Source: CAD feature listing. Evaluate the final solid. Frame: model axes, mm. Face numbers are marked on the shaded views. A direction names the side the tool comes from. Coordinates: 2 decimals unless noted, no trailing zeros. Write each loop counter-clockwise with the first axis right and the second up, starting at its lowest first coordinate (ties: lowest second). Pieces come first, ordered by that corner, then holes. Notation, with made-up numbers: (-8.75, 38) - (15.25, 38) arc R25 ccw to (15.25, 54) - close; hole circle Ø6 at (18, 0.5). An arc over 180 degrees is marked (long way). One line per item, written item: value.
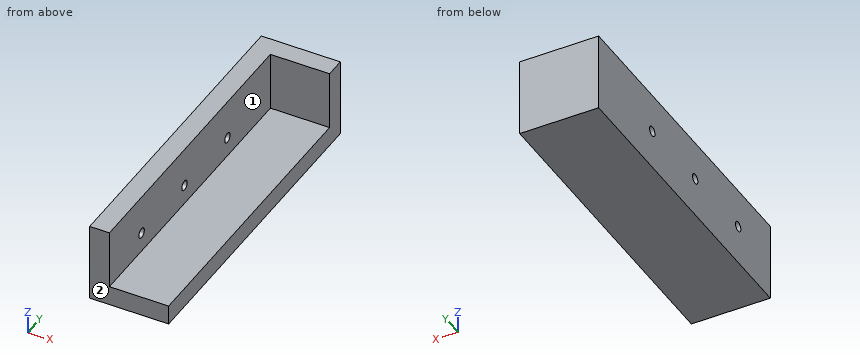
from build123d import *

# Parameters (mm, degrees)
F1_DEPTH = 101.6
F2_W     = 25.4
F2_H     = 25.4
F3_DEPTH = 6.35
F4_R     = 1.5875
F5_DEPTH = 25.4


with BuildPart() as f1:
    # F0 (on Front) → F1 (new body)
    with BuildSketch(Plane.XZ):
        Polygon((0, 25.4), (0, 0), (25.4, 0), (25.4, 6.35), (6.35, 6.35), (6.35, 25.4), align=None)
    extrude(amount=F1_DEPTH)

    # F2 (on Front) → F3 (join)
    with BuildSketch(Plane.XZ):
        with Locations((12.7, 12.7)):
            Rectangle(F2_W, F2_H)
    extrude(amount=F3_DEPTH)

    # F4 (on face) → F5 (cut)
    with BuildSketch(Plane.YZ.offset(6.35)):
        with Locations((-31.75, 12.7)):
            Circle(F4_R)
        with Locations((-57.15, 12.7)):
            Circle(F4_R)
        with Locations((-82.55, 12.7)):
            Circle(F4_R)
    extrude(amount=-F5_DEPTH, mode=Mode.SUBTRACT)


solid = f1.part
1) Reachability of the marked faces 1 and 2 from +Z, -Z, +X, -X, +Y, -Y: full face, straight path, thin tool, end or side. Return the list, or none.
Values found:
face 1: +Z, +X, -Y
face 2: +Z, -Z, +X, -X, -Y
2) Section query C-C on x = 10. Output: boundary loops of the cut face in (y, z).
Values found:
outline: (-101.6, 0) - (0, 0) - (0, 25.4) - (-6.35, 25.4) - (-6.35, 6.35) - (-101.6, 6.35) - close
3) Section query D-D on y = -72. Output: boundary loops of the cut face in (x, z), then the cut area to 3 significant figures.
Values found:
outline: (0, 0) - (25.4, 0) - (25.4, 6.35) - (6.35, 6.35) - (6.35, 25.4) - (0, 25.4) - close
area: 282 mm2
4) Material intervals for line 1 (Z direction, x = 1.5, y = -82.55); line 2 (Y direction, x = 1.5, z = 13.5); line 3 (X direction, y = -14.5, z = 11.75), sorted ascending.
Values found:
line 1: 0 to 11.11, 14.29 to 25.4
line 2: -101.6 to -83.92, -81.18 to -58.52, -55.78 to -33.12, -30.38 to 0
line 3: 0 to 6.35
5) Contact query for flat-ended pins moving along their axis: P1, Ø9.5, axis at y = -45.5, z = 18, coming from the +X side; P2, Ø1.9, axis at y = -82.55, z = 12.7, coming from the +X side; P3, Ø15, axis at x = 14, y = -57.5, coming from the +Z side. Output: stop coordinate, or through.
Values found:
P1: x = 6.35
P2: through
P3: z = 6.35
6) Section query A-A on z = 12.7. Output: boundary loops of the cut face in (x, y), then the cut area to 3 significant figures.
Values found:
outline: (0, -101.6) - (6.35, -101.6) - (6.35, -84.14) - (0, -84.14) - close; (0, -80.96) - (6.35, -80.96) - (6.35, -58.74) - (0, -58.74) - close; (0, -55.56) - (6.35, -55.56) - (6.35, -33.34) - (0, -33.34) - close; (0, -30.16) - (6.35, -30.16) - (6.35, -6.35) - (25.4, -6.35) - (25.4, 0) - (0, 0) - close
area: 706 mm2
7) Section query B-B on y = -31.75. Output: boundary loops of the cut face in (x, z).
Values found:
outline: (0, 0) - (25.4, 0) - (25.4, 6.35) - (6.35, 6.35) - (6.35, 11.11) - (0, 11.11) - close; (0, 14.29) - (6.35, 14.29) - (6.35, 25.4) - (0, 25.4) - close
